Could you check a few things on this model? Use its own coordinates, in mm. A direction names the side the tool comes from. Give positions to 0.01 mm unless a question says otherwise; leave off trailing zeros. Order: outer loops, then holes, each group sorted by start corner. A loop starts at its lowest first (then second) coordinate and runs counter-clockwise, first axis right, second up. Notation, with made-up numbers: M 76,-35 L 95,-35 A18 ccw 95,-22 Z; hole C 22,81 d7. An arc over 180 degrees is marked long. Use a Markdown table: item, result. Add a question column.
Item 1: For faces 4 (the face through (-115.991, -814, 52)), 5 (the face through (-117.254, -814, 51)), which set-ups out of +Z, -Z, +X, -X, +Y, -Y let a thin tool reach every point of the face, with its end or its side?
Item 2: Suppose I cut it at C-C on z = 37. Write out the boundary of the cut face in (x, y), plus the area to 3 significant figures.
Item 3: Suppose I cut it at A-A on y = -798. Write out the boundary of the cut face in (x, z).
Item 4: If we mould it in two halves opening along Z, with no side actions, what happens to faces 1 (the face through (-80, -814, 89.575)), 2 (the face through (-80, -814, 14.655)), 3 (the face through (-41.054, -814, 51))? For each: released by +Z, released by -Z, zero draft, split by the parting line, or undercut.
Item 5: Suppose I cut it at B-B on x = -87. Write out the boundary of the cut face in (y, z).
Item 6: If I drill on L1, parallel to X at y = -750.5, z = 62.5; L2, parallel to Z at x = -106.5, y = -750.5, over which ranges is the centre line in solid material (lowest first)? Write a range as from..to.
from build123d import *

# Parameters (mm, degrees)
F0_W     = 76.2
F0_H     = 76.2
F1_DEPTH = 609.6
F3_DEPTH = 914.4
F4_DEPTH = 304.8
F5_DEPTH = 508
F6_DEPTH = 381
F7_DEPTH = 177.8


with BuildPart() as f1:
    # F0 (on Front) → F1 (new body)
    with BuildSketch(Plane.XZ):
        with Locations((-79.1539917648, 51.4746750653)):
            Rectangle(F0_W, F0_H)
    extrude(amount=F1_DEPTH)

    # F2 (on face) → F3 (cut)
    with BuildSketch(Plane.XZ.offset(609.6)):
        Polygon((-42.3204526305, 88.3055701852), (-98.6881405115, 88.3055701852), (-115.9909814596, 88.3055701852), (-115.9909814596, 14.655277133), (-42.3204526305, 14.655277133), align=None)
    extrude(amount=-F3_DEPTH, mode=Mode.SUBTRACT)

    # F4 (add): a face of the model
    f4_faces = [f1.faces().sort_by_distance(p)[0] for p in [
        (-42.1316224993, -609.6, 51.4746750653),
    ]]
    extrude(f4_faces, amount=F4_DEPTH)

    # F5 (cut): a face of the model
    f5_faces = [f1.faces().sort_by_distance(p)[0] for p in [
        (-42.1316224993, 0, 51.4746750653),
    ]]
    extrude(f5_faces, amount=-F5_DEPTH, mode=Mode.SUBTRACT)

    # F6 (cut): a face of the model
    f6_faces = [f1.faces().sort_by_distance(p)[0] for p in [
        (-42.1316224993, -508, 51.4746750653),
    ]]
    extrude(f6_faces, amount=-F6_DEPTH, mode=Mode.SUBTRACT)

    # F7 (add): a face of the model
    f7_faces = [f1.faces().sort_by_distance(p)[0] for p in [
        (-42.1316224993, -889, 51.4746750653),
    ]]
    extrude(f7_faces, amount=F7_DEPTH)


solid = f1.part
Findings below:
| question | item | result |
|---|---|---|
| 1 | face 4 | +Y, -Y |
| 1 | face 5 | +Z, -Z, -X, +Y, -Y |
| 2 | outline | M -117.25,-914.4 L -115.99,-914.4 L -115.99,-711.2 L -117.25,-711.2 Z; M -42.32,-914.4 L -41.05,-914.4 L -41.05,-711.2 L -42.32,-711.2 Z |
| 2 | area | 514 mm^2 |
| 3 | outline | M -117.25,13.37 L -41.05,13.37 L -41.05,89.57 L -117.25,89.57 Z; hole M -115.99,14.66 L -42.32,14.66 L -42.32,88.31 L -115.99,88.31 Z |
| 4 | face 1 | released by +Z |
| 4 | face 2 | undercut |
| 4 | face 3 | zero draft |
| 5 | outline | M -914.4,13.37 L -711.2,13.37 L -711.2,14.66 L -914.4,14.66 Z; M -914.4,88.31 L -711.2,88.31 L -711.2,89.57 L -914.4,89.57 Z |
| 6 | L1 | x = -117.25..-115.99, -42.32..-41.05 |
| 6 | L2 | z = 13.37..14.66, 88.31..89.57 |
